The drawing under review shows one solid part. Ordinate dimensions are in mm from its lowest x, y, z. A direction names the side the tool comes from. Round coordinates to 2 decimals unless told otherwise and drop trailing zeros. Order: outer loops, then holes, each group sorted by start corner. A loop starts at its lowest first (then second) coordinate and runs counter-clockwise, first axis right, second up. Notation, with made-up numbers: (-17.75, -34) -> (34.25, -34) arc R36 ccw to (34.25, 0) -> close; hole circle Ø10 at (51, -29). An arc over 180 degrees is marked (long way). Use a Markdown table: item, result. Add a question column.
1) Consider section C-C (y = 9.75). State the section outline as (x, z) points.
2) Clearance check with flat-ended pins moving along their axes: P1, Ø4, axis at x = 6.5, y = 2, coming from the -Z side; P2, Ø7.5, axis at y = 4, z = 4, coming from the +X side (1 decimal); P3, Ø3, axis at y = 15.5, z = 5, coming from the -X side. State where each tip first meets the part, or that it passes through.
3) Consider section A-A (z = 3). State the section outline as (x, y) points, plus the area to 3 significant figures.
4) Consider section B-B (x = 7.5). State the section outline as (y, z) points.
5) Machinability: for the marked faces 1, 2 and 3, which of the approach directions +Z, -Z, +X, -X, +Y, -Y give a long, thin tool a straight path to every point of the face, cutting with its end or side? Answer none if there is none.
6) Consider section D-D (x = 13.5). State the section outline as (y, z) points.
7) Wall thickness on line 1 along X through (y, z) = (17.5, 7.25) (1 decimal); line 2 along X through (y, z) = (5, 8.5); line 3 along Y through (x, z) = (2.75, 8.25): over which ranges is each line inside the solid? List them lowest first. Write a range as [from, to].
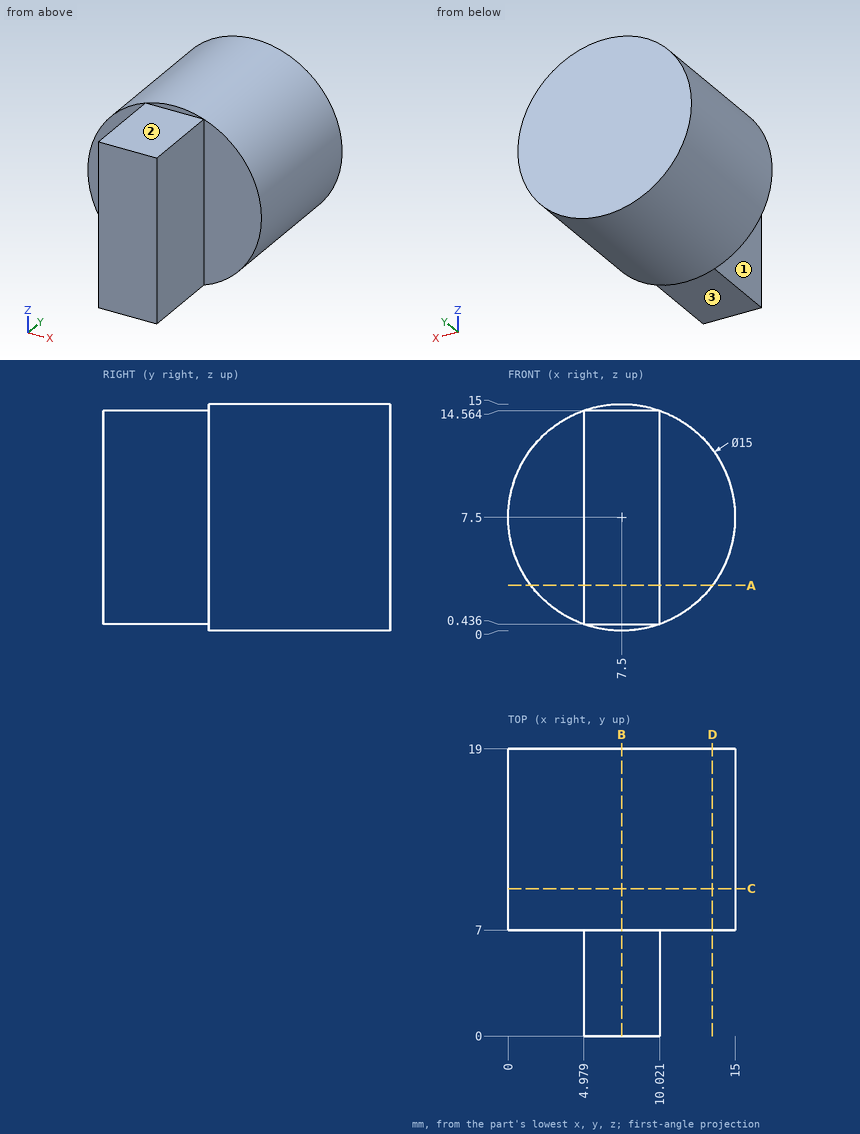
Results list:
| question | item | result |
|---|---|---|
| 1 | outline | circle Ø15 at (7.5, 7.5) |
| 2 | P1 | z = 0.44 |
| 2 | P2 | x = 14.9 |
| 2 | P3 | x = 0.07 |
| 3 | outline | (1.5, 7) -> (4.98, 7) -> (4.98, 0) -> (10.02, 0) -> (10.02, 7) -> (13.5, 7) -> (13.5, 19) -> (1.5, 19) -> close |
| 3 | area | 179 mm2 |
| 4 | outline | (0, 0.44) -> (7, 0.44) -> (7, 0) -> (19, 0) -> (19, 15) -> (7, 15) -> (7, 14.56) -> (0, 14.56) -> close |
| 5 | face 1 | +Z, -Z, -X, -Y |
| 5 | face 2 | +Z, +X, -X, -Y |
| 5 | face 3 | -Z, +X, -X, -Y |
| 6 | outline | (7, 3) -> (19, 3) -> (19, 12) -> (7, 12) -> close |
| 7 | line 1 | [0, 15] |
| 7 | line 2 | [4.98, 10.02] |
| 7 | line 3 | [7, 19] |
